The listing builds one solid part. Answer for the finished solid, in the listing's coordinates (mm). A direction names the side the tool comes from. Round coordinates to 2 decimals unless told otherwise and drop trailing zeros. Write each loop counter-clockwise with the first axis right and the second up, starting at its lowest first coordinate (ties: lowest second). Pieces come first, ordered by that corner, then holes. Notation, with made-up numbers: (-21.75, 12) - (-6.75, 12) arc R13 ccw to (-6.75, 18) - close; hole circle Ø8 at (17.5, -2). An arc over 180 degrees is marked (long way). Answer as CSV lines item,"result". Start each with the question number.
Item 1: Flat-ended cylindrical pins translate along their axes: pin 1 (1.3 mm diameter, centred on x = 0, y = -12, fed in from +Z); pin 2 (2.5 mm diameter, centred on x = 0, y = 12.5, fed in from -Z); pin 3 (3.5 mm diameter, centred on x = 0, y = -12.5, fed in from +Z); pin 4 (1.5 mm diameter, centred on y = -14, z = 10.5, fed in from -X). Find the tip coordinate at first contact, or state that the pin passes through.
Item 2: A cutting plane is placed at C-C on x = 0. Determine the outline of the cut face in (y, z), and give its area (3 significant figures).
Item 3: Straight lines are drawn through the part: line 1 along Y through (x, z) = (0, 62); line 2 along Z through (x, y) = (-5.5, -5); line 3 along Y through (x, z) = (9, 40.5). For each, find the intervals that lie inside material, in ascending order. Write a range as [from, to].
Item 4: A cutting plane is placed at D-D on z = 29. Determine the outline of the cut face in (x, y), and give its area (3 significant figures).
Item 5: Which of the six approach directions +Z, -Z, +X, -X, +Y, -Y give full straight-line access (tool end or side, diameter ignored) to faces 1 (the cylindrical face through (6.018, -2.495, 65.66)), 2 (the flat face through (0, 0, 84.061))?
Item 6: A cutting plane is placed at A-A on y = 0. Determine the outline of the cut face in (x, z), and give its area (3 significant figures).
Item 7: For a pull along Y with two mould halves and no side action, classify faces 3 (the cylindrical face through (-0.34, -1.55, 75.86)), 4 (the flat face through (0, -12, 57.15)), 5 (the flat face through (1.4, -1.4, 67.882)) as pulls with the +Y half, pulls with the -Y half, needs draft (parallel to the pull), parting line crosses it, or undercut.
Item 8: A cutting plane is placed at B-B on z = 61.5. Determine the outline of the cut face in (x, y), and give its area (3 significant figures).
```python
from build123d import *

# Parameters (mm, degrees)
SKETCH1_R           = 19.05
BOSS_EXTRUDE1_DEPTH = 63.5
SKETCH2_R           = 6.5151
BOSS_EXTRUDE2_DEPTH = 4.3815
SKETCH3_R           = 1.5875
BOSS_EXTRUDE3_DEPTH = 16.1798
SKETCH4_R           = 1.27
CUT_EXTRUDE1_DEPTH  = 6.35


with BuildPart() as part:
    # Sketch1 → Boss-Extrude1 (new body)
    with BuildSketch(Plane.XY):
        Circle(SKETCH1_R)
    extrude(amount=BOSS_EXTRUDE1_DEPTH)

    # Sketch2 → Boss-Extrude2 (add)
    with BuildSketch(Plane.XY.offset(63.5)):
        Circle(SKETCH2_R)
    extrude(amount=BOSS_EXTRUDE2_DEPTH)

    # Sketch3 → Boss-Extrude3 (add)
    with BuildSketch(Plane.XY.offset(67.8815)):
        Circle(SKETCH3_R)
    extrude(amount=BOSS_EXTRUDE3_DEPTH)

    # Sketch4 → Cut-Extrude1 (cut)
    with BuildSketch(Plane.XY.offset(63.5)):
        with Locations((0, 12.5)):
            Circle(SKETCH4_R)
        with Locations((0, -12.5)):
            Circle(SKETCH4_R)
    extrude(amount=-CUT_EXTRUDE1_DEPTH, mode=Mode.SUBTRACT)


solid = part.part
```
Geometry says:
1,pin 1,"stops at z = 57.15"
1,pin 2,"stops at z = 0"
1,pin 3,"stops at z = 63.5"
1,pin 4,"stops at x = -13.69"
2,outline,"(-19.05, 0) - (19.05, 0) - (19.05, 63.5) - (13.77, 63.5) - (13.77, 57.15) - (11.23, 57.15) - (11.23, 63.5) - (6.52, 63.5) - (6.52, 67.88) - (1.59, 67.88) - (1.59, 84.06) - (-1.59, 84.06) - (-1.59, 67.88) - (-6.52, 67.88) - (-6.52, 63.5) - (-11.23, 63.5) - (-11.23, 57.15) - (-13.77, 57.15) - (-13.77, 63.5) - (-19.05, 63.5) - close"
2,area,"2,500 mm^2"
3,line 1,"y = [-19.05, -13.77], [-11.23, 11.23], [13.77, 19.05]"
3,line 2,"z = [0, 63.5]"
3,line 3,"y = [-16.79, 16.79]"
4,outline,"circle Ø38.1 at (0, 0)"
4,area,"1,140 mm^2"
5,face 1,"+Z"
5,face 2,"+Z, +X, -X, +Y, -Y"
6,outline,"(-19.05, 0) - (19.05, 0) - (19.05, 63.5) - (6.52, 63.5) - (6.52, 67.88) - (1.59, 67.88) - (1.59, 84.06) - (-1.59, 84.06) - (-1.59, 67.88) - (-6.52, 67.88) - (-6.52, 63.5) - (-19.05, 63.5) - close"
6,area,"2,530 mm^2"
7,face 3,"parting line crosses it"
7,face 4,"undercut"
7,face 5,"needs draft"
8,outline,"circle Ø38.1 at (0, 0); hole circle Ø2.54 at (0, -12.5); hole circle Ø2.54 at (0, 12.5)"
8,area,"1,130 mm^2"
